Read the model definition and answer for the solid it produces. Units are mm, in the model's axes. Face numbers are marked on the shaded views. A direction names the side the tool comes from. Round coordinates to 2 decimals unless told otherwise and drop trailing zeros. Order: outer loops, then holes, each group sorted by start corner. A loop starts at its lowest first (then second) coordinate and runs counter-clockwise, first axis right, second up.
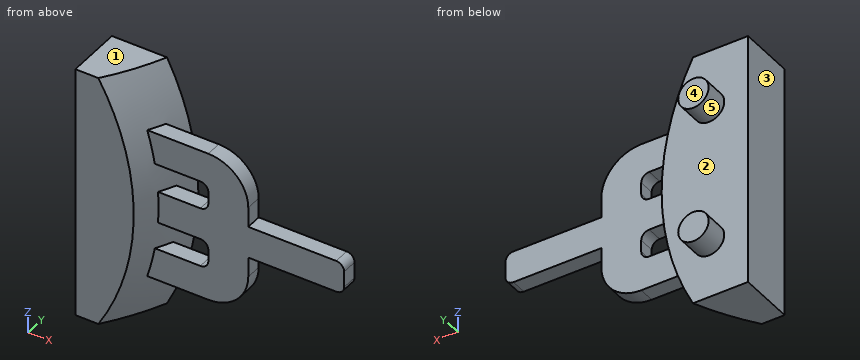
from build123d import *
from build123d.topology import SkipClean

# Parameters (mm, degrees)
CUT_EXTRUDE_3_DEPTH       = 80
CUT_EXTRUDE_START         = -57
CUT_EXTRUDE_4_DEPTH       = 57
CUT_EXTRUDE_4_2_OUTLINE_W = 14.17
CUT_EXTRUDE_4_2_OUTLINE_H = 32
CUT_EXTRUDE_4_2_DEPTH     = 50
SKETCH_7_R                = 1.9
EXTRUDE_2_DEPTH           = 3
SKETCH_8_W                = 4
SKETCH_8_H                = 2
EXTRUDE_3_DEPTH           = 15
SKETCH_9_W                = 19
SKETCH_9_H                = 2
EXTRUDE_4_DEPTH           = 5
SKETCH_8_2_W              = 4
SKETCH_8_2_H              = 2
EXTRUDE_5_DEPTH           = 32
FILLET_1_R                = 5
FILLET_2_R                = 1
FILLET_3_R                = 1


# Read off the part's stored shape, not the designer's step: 컷-돌출4
with BuildPart() as part:
    # 스케치4 → 회전1 (revolve)
    with SkipClean():  # the faces are left unmerged after this step: merging them gives an invalid solid
        with BuildSketch(Plane.XY):
            with BuildLine():
                ThreePointArc((37, 0), (26.162950904, 26.162950904), (0, 37))
                Line((0, 37), (0, -37))
                ThreePointArc((0, -37), (26.162950904, -26.162950904), (37, 0))
            make_face()
            with BuildLine():
                Line((0, -37), (0, 37))
                ThreePointArc((0, 37), (-37, 0), (0, -37))
            make_face()
        revolve(axis=Axis((0, 48.172126022, 0), (0, -1, 0)))

    # 스케치5 → 컷-돌출3 (cut, symmetric)
    with SkipClean():  # the faces are left unmerged after this step: merging them gives an invalid solid
        with BuildSketch(Plane.XY):
            Polygon((-37.71852549, -20), (40.89907451, -20), (49.098598746, -47.851019931), (-38.951742745, -43.163184314), align=None)
        extrude(amount=CUT_EXTRUDE_3_DEPTH, both=True, mode=Mode.SUBTRACT)

    # 컷-돌출4 outline → 컷-돌출4 (cut)
    with BuildSketch(Plane.XZ.offset(20).offset(CUT_EXTRUDE_START)):
        Polygon((23.83, -16), (23.83, 16), (38, 16), (38, 38), (-38, 38), (-38, -38), (38, -38), (38, -16), align=None)
    extrude(amount=CUT_EXTRUDE_4_DEPTH, mode=Mode.SUBTRACT)

    # Cut-Extrude 4 2 outline → Cut-Extrude 4 2 (cut)
    with BuildSketch(Plane.XZ.offset(20).offset(CUT_EXTRUDE_START)):
        with Locations((30.915, 0)):
            Rectangle(CUT_EXTRUDE_4_2_OUTLINE_W, CUT_EXTRUDE_4_2_OUTLINE_H)
    extrude(amount=CUT_EXTRUDE_4_2_DEPTH, mode=Mode.SUBTRACT)

    # 스케치7 → 보스-돌출2 (add)
    with BuildSketch(Plane(origin=(0, -13, 0), x_dir=(1, 0, 0), z_dir=(0, 1, 0))):
        with Locations(Location((28.71, 8.68, 0), (0, 0, 90))):
            Circle(SKETCH_7_R)
        with Locations(Location((28.71, -8.68, 0), (0, 0, 90))):
            Circle(SKETCH_7_R)
    extrude(amount=EXTRUDE_2_DEPTH)

    # 스케치8 → 보스-돌출3 (add)
    with BuildSketch(Plane.ZY.offset(-23.83)):
        with Locations((-7.5, -16.5)):
            Rectangle(SKETCH_8_W, SKETCH_8_H)
        with Locations((0, -16.5)):
            Rectangle(SKETCH_8_W, SKETCH_8_H)
        with Locations((7.5, -16.5)):
            Rectangle(SKETCH_8_W, SKETCH_8_H)
    extrude(amount=-EXTRUDE_3_DEPTH)

    # 스케치9 → 보스-돌출4 (add)
    with BuildSketch(Plane(origin=(38.83, 0, 0), x_dir=(0, 0, -1), z_dir=(1, 0, 0))):
        with Locations((0, -16.5)):
            Rectangle(SKETCH_9_W, SKETCH_9_H)
    extrude(amount=EXTRUDE_4_DEPTH)

    # 스케치8<2> → 보스-돌출5 (add)
    with BuildSketch(Plane.ZY.offset(-23.83)):
        with Locations((0, -16.5)):
            Rectangle(SKETCH_8_2_W, SKETCH_8_2_H)
    extrude(amount=-EXTRUDE_5_DEPTH)

    # 필렛1
    fillet_1_edges = [part.edges().sort_by_distance(p)[0] for p in [
        (43.83, -16.5, 9.5),
        (43.83, -16.5, -9.5),
    ]]
    fillet(fillet_1_edges, radius=FILLET_1_R)

    # 필렛2
    fillet_2_edges = [part.edges().sort_by_distance(p)[0] for p in [
        (38.83, -16.5, 2),
        (38.83, -16.5, -2),
        (38.83, -16.5, 5.5),
        (38.83, -16.5, -5.5),
    ]]
    fillet(fillet_2_edges, radius=FILLET_2_R)

    # 필렛3
    fillet_3_edges = [part.edges().sort_by_distance(p)[0] for p in [
        (55.83, -16.5, 2),
        (55.83, -16.5, -2),
    ]]
    fillet(fillet_3_edges, radius=FILLET_3_R)


solid = part.part
Q1. Flat-ended cylindrical pins translate along their axes: pin 1 (1 mm diameter, centred on x = 35.5, y = -16.5, fed in from +Z); pin 2 (0.6 mm diameter, centred on x = 35.5, y = -16, fed in from -Z); pin 3 (1 mm diameter, centred on y = -16, z = -3, fed in from +X); pin 4 (5 mm diameter, centred on x = 29, z = 12, fed in from -Y). Find the tip coordinate at first contact, or state that the pin passes through.
Outcome:
pin 1: stops at z = 9.5
pin 2: stops at z = -9.5
pin 3: stops at x = 43.83
pin 4: stops at y = -20
Q2. For a pull along Z with two mould halves and no side action, classify the marked faces 1, 2 and 3 as released by +Z, released by -Z, zero draft, split by the parting line, or undercut.
Outcome:
face 1: released by +Z
face 2: undercut
face 3: zero draft
Q3. A cutting plane is placed at B-B, the plane z = 10. Give the vertices of the cut face in (x, y), plus the area to 3 significant figures.
Outcome:
outline: (23.83, -20) - (29.48, -20) arc R35.62 ccw to (33.17, -13) - (30.08, -13) - (30.08, -10) - (27.34, -10) - (27.34, -13) - (23.83, -13) - close
area: 61.8 mm2
Q4. Straight lines are drawn through the part: probe 1 along Y at (x, z) = (39, -4.5); probe 2 along Y at (x, z) = (27, 4.5); probe 3 along X at (y, z) = (-17, -4). For each, find the intervals that lie inside material, in ascending order.
Outcome:
probe 1: y = -17.5 to -15.5
probe 2: y = -20 to -13
probe 3: x = 23.83 to 32.62, 38.83 to 43.83
Q5. For the marked faces 4 and 5, determine the directions among +Z, -Z, +X, -X, +Y, -Y from which every point of the face is accessible in a straight line to the end or side of a thin tool.
Outcome:
face 4: +Z, -Z, +X, -X, +Y
face 5: +Y
Q6. A cutting plane is placed at A-A, the plane y = -16.25. Give the vertices of the cut face in (x, z), plus the area to 3 significant figures.
Outcome:
outline: (23.83, -16) - (29.14, -16) arc R33.24 ccw to (31.85, -9.5) - (38.83, -9.5) arc R5 ccw to (43.83, -4.5) - (43.83, -2) - (54.83, -2) arc R1 ccw to (55.83, -1) - (55.83, 1) arc R1 ccw to (54.83, 2) - (43.83, 2) - (43.83, 4.5) arc R5 ccw to (38.83, 9.5) - (31.85, 9.5) arc R33.24 ccw to (29.14, 16) - (23.83, 16) - close; hole (32.78, -5.5) - (37.83, -5.5) arc R1 ccw to (38.83, -4.5) - (38.83, -3) arc R1 ccw to (37.83, -2) - (33.18, -2) arc R33.24 cw to start; hole (32.78, 5.5) arc R33.24 cw to (33.18, 2) - (37.83, 2) arc R1 ccw to (38.83, 3) - (38.83, 4.5) arc R1 ccw to (37.83, 5.5) - close
area: 465 mm2
Q7. A cutting plane is placed at C-C, the plane y = -11.5. Give the vertices of the cut face in (x, z), plus the area to 3 significant figures.
Outcome:
outline: circle Ø3.8 at (28.71, -8.68); circle Ø3.8 at (28.71, 8.68)
area: 22.7 mm2
Q8. A cutting plane is placed at D-D, the plane x = 45. Give the vertices of the cut face in (y, z).
Outcome:
outline: (-17.5, -2) - (-15.5, -2) - (-15.5, 2) - (-17.5, 2) - close
